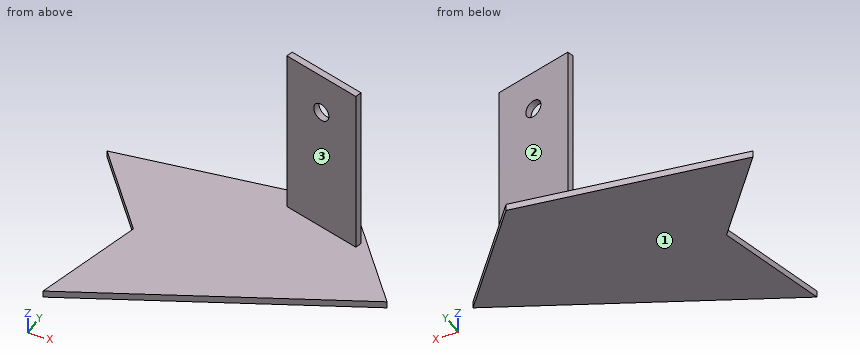
Autodesk Inventor part; units mm, degrees
ref_plane "YZ Plane" through (0, 0, 0) normal (1, 0, 0) x (0, 1, 0)
ref_plane "XZ Plane" through (0, 0, 0) normal (0, 1, 0) x (-1, 0, 0)
ref_plane "XY Plane" through (0, 0, 0) normal (0, 0, 1) x (1, 0, 0)
sketch "Sketch1" plane through (0, 0, 0) normal (0, 0, 1) x (1, 0, 0)
  line L0 (-10.4788, 3.5567) -> (22.1748, -35.3584)
  line L1 (-10.4788, 3.5567) -> (40.3212, 3.5567) construction
  line L2 (22.1748, -35.3584) -> (8.205, -87.4942)
  line L3 (8.205, -87.4942) -> (134.8162, -28.4545)
  line L4 (134.8162, -28.4545) -> (93.9992, 20.1894)
  line L5 (93.9992, 20.1894) -> (-10.4788, 3.5567)
  point P0 (0, 0)
  dimension "d0" = 50.8
  dimension "d1" = 50
  dimension "d2" = 53.975
  dimension "d3" = 125
  dimension "d4" = 139.7
  dimension "d5" = 50
  dimension "d6" = 63.5
  dimension "d7" = 75
extrude "Extrusion1" add sketch "Sketch1" along normal blind 3.175
sketch "Sketch2" plane through (0, 0, 3.175) normal (0, 0, 1) x (1, 0, 0)
  line L0 (22.1748, -35.3584) -> (8.205, -87.4942)
  line L1 (8.205, -87.4942) -> (8.205, -87.4942)
  line L2 (93.9992, 20.1894) -> (113.481, 20.1894) construction
  line L3 (88.957, 1.3714) -> (107.3579, -3.5591)
  line L4 (107.3579, -3.5591) -> (108.1796, -0.4923)
  line L5 (108.1796, -0.4923) -> (71.3778, 9.3687)
  line L6 (71.3778, 9.3687) -> (70.5561, 6.3019)
  line L7 (88.957, 1.3714) -> (70.5561, 6.3019)
  point P0 (0, 0)
  dimension "d10" = 19.4818
  dimension "d12" = 19.05
  dimension "d13" = 3.175
  dimension "d14" = 38.1
extrude "Extrusion2" add sketch "Sketch2" along normal blind 79.2734
sketch "Sketch3" plane through (71.3778, 9.3687, 82.4484) normal (0.2588, 0.9659, 0) x (0.9659, -0.2588, 0)
  line L0 (0, 0) -> (19.05, 0)
  line L1 (19.05, 0) -> (19.05, 19.05)
  line L2 (19.05, 19.05) -> (0, 19.05)
  line L3 (0, 19.05) -> (0, 0)
  point P0 (-66.5209, 82.4484)
  dimension "d17" = 19.05
  dimension "d18" = 19.05
hole "Hole1" at (89.7787, 4.4382, 63.3984) direction (-0.2588, -0.9659, 0) diameter 8.3312 end through all
properties part number "Left Bicep"
The listing builds one solid part. Answer for the finished solid, in the listing's coordinates (mm). Face numbers are marked on the shaded views. A direction names the side the tool comes from. Coordinates: 2 decimals unless noted, no trailing zeros. Write each loop counter-clockwise with the first axis right and the second up, starting at its lowest first coordinate (ties: lowest second). Pieces come first, ordered by that corner, then holes. Notation, with made-up numbers: M -24.5,61 L -9.5,61 A25 ccw -9.5,93 Z; hole C 31,70 d6. An arc over 180 degrees is marked long. Use a Markdown table: item, result. Add a question column.
1. Given P1, Ø1, axis at x = 119, y = -14.5, coming from the +Z side (3 decimals); P2, Ø6, axis at y = -5.5, z = 33.5, coming from the +X side; P3, Ø2, axis at x = 91, z = 46.5, coming from the +Y side, each flat-ended and moving along its own axis, determine where each tip first touches the part or whether it passes through.
2. Section C-C (x = 98) is taken. Give the vertices of the cut face in (y, z) (3 decimals).
3. Straight lines are drawn through the part: line 1 along Z through (x, y) = (28, -67) (3 decimals); line 2 along Y through (x, z) = (75, 54.5); line 3 along Y through (x, z) = (88, 21). For each, find the intervals that lie inside material, in ascending order. Write a range as [from, to].
4. Section D-D (y = -8) is taken. Give the vertices of the cut face in (x, z) (3 decimals), plus the area to 3 significant figures.
5. Which of the six approach directions +Z, -Z, +X, -X, +Y, -Y give full straight-line access (tool end or side, diameter ignored) to the marked faces 1, 2 and 3?
6. Section B-B (z = 17) is taken. Give the vertices of the cut face in (x, y), plus the area to 3 significant figures.
7. Section A-A (x = 20) is taken. Give the vertices of the cut face in (y, z) (3 decimals).
Data:
| question | item | result |
|---|---|---|
| 1 | P1 | stops at z = 3.175 |
| 1 | P2 | stops at x = 107.64 |
| 1 | P3 | stops at y = 4.38 |
| 2 | outline | M -45.622,0 L 15.421,0 L 15.421,3.175 L 2.235,3.175 L 2.235,82.448 L -1.052,82.448 L -1.052,3.175 L -45.622,3.175 Z |
| 3 | line 1 | z = [0, 3.175] |
| 3 | line 2 | y = [5.11, 8.4] |
| 3 | line 3 | y = [1.63, 4.91] |
| 4 | outline | M -0.782,0 L 117.653,0 L 117.653,3.175 L -0.782,3.175 Z |
| 4 | area | 376 mm2 |
| 5 | face 1 | -Z, +X, -X, +Y, -Y |
| 5 | face 2 | +Z, +X, +Y |
| 5 | face 3 | +Z, -X, -Y |
| 6 | outline | M 70.56,6.3 L 107.36,-3.56 L 108.18,-0.49 L 71.38,9.37 Z |
| 6 | area | 121 mm2 |
| 7 | outline | M -81.994,0 L -43.475,0 L -43.475,3.175 L -81.994,3.175 Z; M -32.767,0 L 8.409,0 L 8.409,3.175 L -32.767,3.175 Z |
